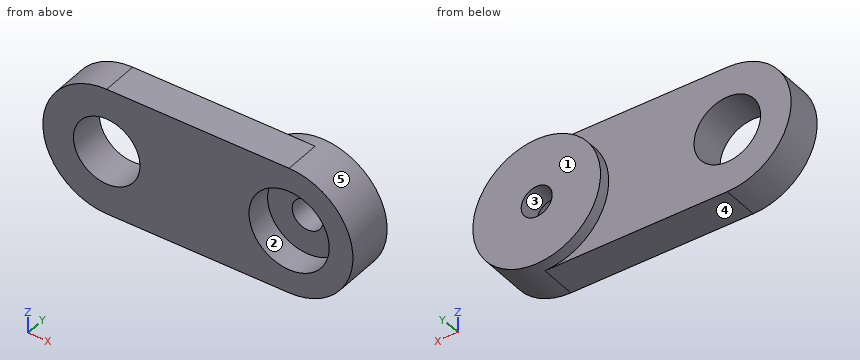
```python
from build123d import *

# Parameters (mm, degrees)
SKETCH1_R             = 2.31775
SKETCH1_R_2           = 1.0795
BASE_EXTRUDE_DEPTH    = 2.54
SKETCH2_R             = 4.445
SKETCH2_R_2           = 1.0795
SERVO_EXTRUDE_DEPTH   = 0.8
SKETCH3_R             = 2.794
SKETCH3_R_2           = 1.0795
SERVO_MOUNT_CUT_DEPTH = 1.816


with BuildPart() as part:
    # Sketch1 → Base Extrude (new body)
    with BuildSketch(Plane(origin=(0, 0, 0), x_dir=(1, 0, 0), z_dir=(0, 1, 0))):
        with BuildLine():
            ThreePointArc((0, 4.445), (-4.445, 0), (0, -4.445))
            Line((0, -4.445), (12.7, -4.445))
            ThreePointArc((12.7, -4.445), (17.145, 0), (12.7, 4.445))
            Line((12.7, 4.445), (0, 4.445))
        make_face()
        with Locations(Location((0, 0, 0), (0, 0, 270))):
            Circle(SKETCH1_R, mode=Mode.SUBTRACT)
        with Locations(Location((12.7, 0, 0), (0, 0, 270))):
            Circle(SKETCH1_R_2, mode=Mode.SUBTRACT)
    extrude(amount=BASE_EXTRUDE_DEPTH)

    # Sketch2 → Servo Extrude (add)
    with BuildSketch(Plane(origin=(0, 2.54, 0), x_dir=(1, 0, 0), z_dir=(0, 1, 0))):
        with Locations(Location((12.7, 0, 0), (0, 0, 270))):
            Circle(SKETCH2_R)
        with Locations(Location((12.7, 0, 0), (0, 0, 270))):
            Circle(SKETCH2_R_2, mode=Mode.SUBTRACT)
    extrude(amount=SERVO_EXTRUDE_DEPTH)

    # Sketch3 → Servo Mount Cut (cut)
    with BuildSketch(Plane.XZ):
        with Locations(Location((12.7, 0, 0), (0, 0, 270))):
            Circle(SKETCH3_R)
        with Locations(Location((12.7, 0, 0), (0, 0, 90))):
            Circle(SKETCH3_R_2, mode=Mode.SUBTRACT)
    extrude(amount=-SERVO_MOUNT_CUT_DEPTH, mode=Mode.SUBTRACT)


solid = part.part
```
Here's how the part is built. I have some questions about the finished solid (model axes, mm). Face numbers are marked on the shaded views. A direction names the side the tool comes from. Give positions to 0.01 mm unless a question says otherwise; leave off trailing zeros. Order: outer loops, then holes, each group sorted by start corner. A loop starts at its lowest first (then second) coordinate and runs counter-clockwise, first axis right, second up. Notation, with made-up numbers: (0, -32.75) - (23, -32.75) arc R23 ccw to (23, -9.75) - close; hole circle Ø4 at (76, 50). An arc over 180 degrees is marked (long way). Answer as a JSON object with one key per item and string values. Group by question number.
Item 1: For P1, Ø5, axis at x = 3.5, z = 2.5, coming from the +Y side; P2, Ø1, axis at y = 2, z = 2.5, coming from the -X side, each with a flat end and sliding along its axis, tell me the tip position at first contact or that it passes through.
Item 2: If we section it at A-A on z = 0: Please give me the cut outline in (x, y) (1 decimal), and give its area (3 significant figures).
Item 3: Please list where these lines run through material, in increasing order: probe 1 along X at (y, z) = (0.6, 0) (3 decimals); probe 2 along X at (y, z) = (2.2, 0) (1 decimal); probe 3 along Z at (x, y) = (12.7, 2.7) (1 decimal).
Item 4: If we section it at C-C on z = -1.5: Please give me the cut outline in (x, y).
Item 5: If we section it at D-D on x = 9: Please give me the cut outline in (y, z) (3 decimals).
Item 6: If we mould it in two halves opening along Z, with no side actions, what happens to the marked faces 3, 4 and 5? For each: pulls with the +Z half, pulls with the -Z half, needs draft (parallel to the pull), parting line crosses it, or undercut.
Item 7: If we section it at B-B on x = -1.5: Please give me the cut outline in (y, z), and give its area (3 significant figures).
Item 8: Which directions (+Z, -Z, +X, -X, +Y, -Y) give clear straight access to the entire face, cutting with the end or side of a thin tool? Please do the marked faces 1 and 2.
Result set:
{
 "1": {"P1": "y = 2.54", "P2": "x = -3.97"},
 "2": {"outline": "(-4.4, 0) - (-2.3, 0) - (-2.3, 2.5) - (-4.4, 2.5) - close; (2.3, 0) - (9.9, 0) - (9.9, 1.8) - (11.6, 1.8) - (11.6, 3.3) - (8.3, 3.3) - (8.3, 2.5) - (2.3, 2.5) - close; (13.8, 1.8) - (15.5, 1.8) - (15.5, 0) - (17.1, 0) - (17.1, 3.3) - (13.8, 3.3) - close", "area": "36.7 mm²"},
 "3": {"probe 1": "-4.445 to -2.318, 2.318 to 9.906, 15.494 to 17.145", "probe 2": "-4.4 to -2.3, 2.3 to 11.6, 13.8 to 17.1", "probe 3": "-4.4 to -1.1, 1.1 to 4.4"},
 "4": {"outline": "(-4.18, 0) - (-1.77, 0) - (-1.77, 2.54) - (-4.18, 2.54) - close; (1.77, 0) - (10.34, 0) - (10.34, 1.82) - (15.06, 1.82) - (15.06, 0) - (16.88, 0) - (16.88, 3.34) - (8.52, 3.34) - (8.52, 2.54) - (1.77, 2.54) - close"},
 "5": {"outline": "(0, -4.445) - (2.54, -4.445) - (2.54, -2.463) - (3.34, -2.463) - (3.34, 2.463) - (2.54, 2.463) - (2.54, 4.445) - (0, 4.445) - close"},
 "6": {"face 3": "undercut", "face 4": "pulls with the -Z half", "face 5": "parting line crosses it"},
 "7": {"outline": "(0, -4.18) - (2.54, -4.18) - (2.54, -1.77) - (0, -1.77) - close; (0, 1.77) - (2.54, 1.77) - (2.54, 4.18) - (0, 4.18) - close", "area": "12.3 mm²"},
 "8": {"face 1": "+Z, -Z, +X, -X, +Y", "face 2": "-Y"}
}
